Build history of the part. All positions in model axes, mm. Round coordinates to 2 decimals unless told otherwise and drop trailing zeros. One line per question, with ' | ' between items. Start each with the question number.
from build123d import *

# Parameters (mm, degrees)
SKETCH1_W               = 508
SKETCH1_H               = 127
BOSS_EXTRUDE1_DEPTH     = 0.85
CUT_EXTRUDE1_DEPTH      = 262.822726286
CUT_EXTRUDE1_DEPTH_BACK = 262.822726286
FILLET1_R               = 10
SKETCH3_W               = 101.6
SKETCH3_H               = 63.5
CUT_EXTRUDE2_DEPTH      = 262.822726286
FILLET2_R               = 10
SKETCH8_R               = 2.07
CUT_EXTRUDE3_DEPTH      = 1.7
SKETCH12_R              = 3.05
CUT_EXTRUDE4_DEPTH      = 262.822726286


with BuildPart() as part:
    # Sketch1 → Boss-Extrude1 (new, symmetric)
    with BuildSketch(Plane(origin=(0, 0, 0), x_dir=(1, 0, 0), z_dir=(0, 1, 0))):
        Rectangle(SKETCH1_W, SKETCH1_H)
    extrude(amount=BOSS_EXTRUDE1_DEPTH, both=True)

    # Sketch2 → Cut-Extrude1 (cut, two sides: drawn at the far end of the back side and taken through both)
    with BuildSketch(Plane(origin=(0, 0.85, 0), x_dir=(1, 0, 0), z_dir=(0, 1, 0)).offset(-CUT_EXTRUDE1_DEPTH_BACK)):
        with BuildLine():
            Line((251.65, -43.625), (251.65, -51.625))
            ThreePointArc((251.65, -51.625), (247.65, -55.625), (243.65, -51.625))
            Line((243.65, -51.625), (243.65, -43.625))
            ThreePointArc((243.65, -43.625), (247.65, -39.625), (251.65, -43.625))
        make_face()
        with BuildLine():
            Line((251.65, -19.875), (251.65, -11.875))
            ThreePointArc((251.65, -11.875), (247.65, -7.875), (243.65, -11.875))
            Line((243.65, -11.875), (243.65, -19.875))
            ThreePointArc((243.65, -19.875), (247.65, -23.875), (251.65, -19.875))
        make_face()
        with BuildLine():
            Line((251.65, 19.875), (251.65, 11.875))
            ThreePointArc((251.65, 11.875), (247.65, 7.875), (243.65, 11.875))
            Line((243.65, 11.875), (243.65, 19.875))
            ThreePointArc((243.65, 19.875), (247.65, 23.875), (251.65, 19.875))
        make_face()
        with BuildLine():
            Line((251.65, 43.625), (251.65, 51.625))
            ThreePointArc((251.65, 51.625), (247.65, 55.625), (243.65, 51.625))
            Line((243.65, 51.625), (243.65, 43.625))
            ThreePointArc((243.65, 43.625), (247.65, 39.625), (251.65, 43.625))
        make_face()
        with BuildLine():
            Line((-251.65, 43.625), (-251.65, 51.625))
            ThreePointArc((-251.65, 51.625), (-247.65, 55.625), (-243.65, 51.625))
            Line((-243.65, 51.625), (-243.65, 43.625))
            ThreePointArc((-243.65, 43.625), (-247.65, 39.625), (-251.65, 43.625))
        make_face()
        with BuildLine():
            Line((-251.65, 19.875), (-251.65, 11.875))
            ThreePointArc((-251.65, 11.875), (-247.65, 7.875), (-243.65, 11.875))
            Line((-243.65, 11.875), (-243.65, 19.875))
            ThreePointArc((-243.65, 19.875), (-247.65, 23.875), (-251.65, 19.875))
        make_face()
        with BuildLine():
            Line((-251.65, -19.875), (-251.65, -11.875))
            ThreePointArc((-251.65, -11.875), (-247.65, -7.875), (-243.65, -11.875))
            Line((-243.65, -11.875), (-243.65, -19.875))
            ThreePointArc((-243.65, -19.875), (-247.65, -23.875), (-251.65, -19.875))
        make_face()
        with BuildLine():
            Line((-251.65, -43.625), (-251.65, -51.625))
            ThreePointArc((-251.65, -51.625), (-247.65, -55.625), (-243.65, -51.625))
            Line((-243.65, -51.625), (-243.65, -43.625))
            ThreePointArc((-243.65, -43.625), (-247.65, -39.625), (-251.65, -43.625))
        make_face()
    extrude(amount=CUT_EXTRUDE1_DEPTH + CUT_EXTRUDE1_DEPTH_BACK, mode=Mode.SUBTRACT)

    # Fillet1
    fillet1_edges = [part.edges().sort_by_distance(p)[0] for p in [
        (-254, 0, -63.5),
        (254, 0, -63.5),
        (254, 0, 63.5),
        (-254, 0, 63.5),
    ]]
    fillet(fillet1_edges, radius=FILLET1_R)

    # Sketch3 → Cut-Extrude2 (cut, through all)
    with BuildSketch(Plane(origin=(0, 0.85, 0), x_dir=(1, 0, 0), z_dir=(0, 1, 0))):
        with Locations((-25.4, 31.75)):
            Rectangle(SKETCH3_W, SKETCH3_H)
    extrude(amount=-CUT_EXTRUDE2_DEPTH, mode=Mode.SUBTRACT)

    # Fillet2
    fillet2_edges = [part.edges().sort_by_distance(p)[0] for p in [
        (-76.2, 0, 0),
        (-76.2, 0, -63.5),
        (25.4, 0, -63.5),
        (25.4, 0, 0),
    ]]
    fillet(fillet2_edges, radius=FILLET2_R)

    # Sketch8 → Cut-Extrude3 (cut)
    with BuildSketch(Plane(origin=(0, 0.85, 0), x_dir=(1, 0, 0), z_dir=(0, 1, 0))):
        with Locations(Location((-165.1, 0, 0), (0, 0, 270))):
            Circle(SKETCH8_R)
        with Locations(Location((-25.4, -31.75, 0), (0, 0, 270))):
            Circle(SKETCH8_R)
        with Locations(Location((139.7, 0, 0), (0, 0, 270))):
            Circle(SKETCH8_R)
        with Locations(Location((-228.6, -56.5, 0), (0, 0, 270))):
            Circle(SKETCH8_R)
        with Locations(Location((-203.2, -56.5, 0), (0, 0, 270))):
            Circle(SKETCH8_R)
        with Locations(Location((-177.8, -56.5, 0), (0, 0, 270))):
            Circle(SKETCH8_R)
        with Locations(Location((-152.4, -56.5, 0), (0, 0, 270))):
            Circle(SKETCH8_R)
        with Locations(Location((-127, -56.5, 0), (0, 0, 270))):
            Circle(SKETCH8_R)
        with Locations(Location((-101.6, -56.5, 0), (0, 0, 270))):
            Circle(SKETCH8_R)
        with Locations(Location((-76.2, -56.5, 0), (0, 0, 270))):
            Circle(SKETCH8_R)
        with Locations(Location((-50.8, -56.5, 0), (0, 0, 270))):
            Circle(SKETCH8_R)
        with Locations(Location((-25.4, -56.5, 0), (0, 0, 270))):
            Circle(SKETCH8_R)
        with Locations(Location((0, -56.5, 0), (0, 0, 270))):
            Circle(SKETCH8_R)
        with Locations(Location((25.4, -56.5, 0), (0, 0, 270))):
            Circle(SKETCH8_R)
        with Locations(Location((50.8, -56.5, 0), (0, 0, 270))):
            Circle(SKETCH8_R)
        with Locations(Location((76.2, -56.5, 0), (0, 0, 270))):
            Circle(SKETCH8_R)
        with Locations(Location((101.6, -56.5, 0), (0, 0, 270))):
            Circle(SKETCH8_R)
        with Locations(Location((127, -56.5, 0), (0, 0, 270))):
            Circle(SKETCH8_R)
        with Locations(Location((152.4, -56.5, 0), (0, 0, 270))):
            Circle(SKETCH8_R)
        with Locations(Location((177.8, -56.5, 0), (0, 0, 270))):
            Circle(SKETCH8_R)
        with Locations(Location((203.2, -56.5, 0), (0, 0, 270))):
            Circle(SKETCH8_R)
        with Locations(Location((228.6, -56.5, 0), (0, 0, 270))):
            Circle(SKETCH8_R)
        with Locations(Location((-228.6, 56.5, 0), (0, 0, 270))):
            Circle(SKETCH8_R)
        with Locations(Location((-203.2, 56.5, 0), (0, 0, 270))):
            Circle(SKETCH8_R)
        with Locations(Location((-177.8, 56.5, 0), (0, 0, 270))):
            Circle(SKETCH8_R)
        with Locations(Location((-152.4, 56.5, 0), (0, 0, 270))):
            Circle(SKETCH8_R)
        with Locations(Location((-127, 56.5, 0), (0, 0, 270))):
            Circle(SKETCH8_R)
        with Locations(Location((-101.6, 56.5, 0), (0, 0, 270))):
            Circle(SKETCH8_R)
        with Locations(Location((50.8, 56.5, 0), (0, 0, 270))):
            Circle(SKETCH8_R)
        with Locations(Location((76.2, 56.5, 0), (0, 0, 270))):
            Circle(SKETCH8_R)
        with Locations(Location((101.6, 56.5, 0), (0, 0, 270))):
            Circle(SKETCH8_R)
        with Locations(Location((127, 56.5, 0), (0, 0, 270))):
            Circle(SKETCH8_R)
        with Locations(Location((152.4, 56.5, 0), (0, 0, 270))):
            Circle(SKETCH8_R)
        with Locations(Location((177.8, 56.5, 0), (0, 0, 270))):
            Circle(SKETCH8_R)
        with Locations(Location((203.2, 56.5, 0), (0, 0, 270))):
            Circle(SKETCH8_R)
        with Locations(Location((228.6, 56.5, 0), (0, 0, 270))):
            Circle(SKETCH8_R)
    extrude(amount=-CUT_EXTRUDE3_DEPTH, mode=Mode.SUBTRACT)

    # Sketch12 → Cut-Extrude4 (cut, through all)
    with BuildSketch(Plane(origin=(0, 0.85, 0), x_dir=(1, 0, 0), z_dir=(0, 1, 0))):
        with Locations(Location((50.8, 38.1, 0), (0, 0, 270))):
            Circle(SKETCH12_R)
        with Locations(Location((50.8, 3.1, 0), (0, 0, 270))):
            Circle(SKETCH12_R)
        with Locations(Location((50.8, -31.9, 0), (0, 0, 270))):
            Circle(SKETCH12_R)
    extrude(amount=-CUT_EXTRUDE4_DEPTH, mode=Mode.SUBTRACT)


solid = part.part
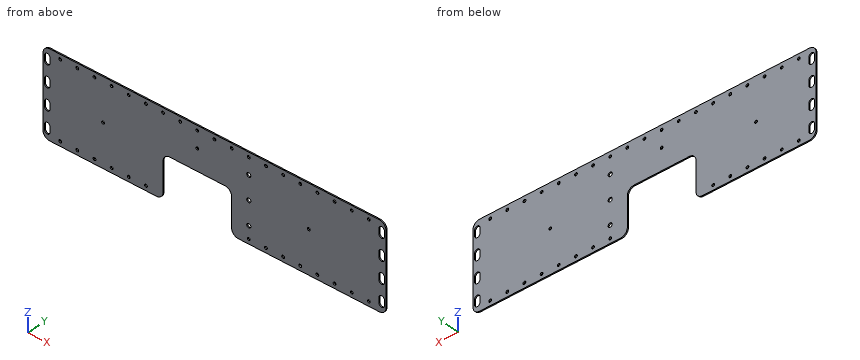
Item 1: Flat gauge pins, fed straight in: pin 1 (3.5 mm diameter, centred on x = -50.8, z = 56.5, fed in from +Y); pin 2 (5 mm diameter, centred on x = 127, z = -56.5, fed in from -Y). Where does each tip first touch, or does it go through?
Item 2: Cut at A-A on y = 0.3. Count the separate pieces of the cut face and the enclosed holes in it, then the cut area to 3 significant figures.
Item 3: Wall check: line 1 along X through (y, z) = (0.8, 20); line 2 along Z through (x, y) = (152.4, 0.35); line 3 along X through (y, z) = (-0.3, 30). Give the ranges that are in metal, low to high. Write a range as [from, to].
Results found:
1) pin 1: passes through | pin 2: stops at y = -0.85
2) separate pieces: 1 | enclosed holes: 47 | area: 56,500 mm^2
3) line 1: x = [-254, -251.65], [-243.65, 243.65], [251.65, 254] | line 2: z = [-63.5, -58.57], [-54.43, 54.43], [58.57, 63.5] | line 3: x = [-254, -26.51], [-24.29, 48.41], [53.19, 254]
